CAD build for the part. Positions are in the model's coordinates, mm. Coordinates: 2 decimals unless noted, no trailing zeros. Loops run counter-clockwise (first coordinate to the right, second up) from the corner with the lowest first, then second, coordinate; pieces in that order, holes last. Notation, with made-up numbers: (-15.75, 58.5) -> (3.25, 58.5) arc R21 cw to (3.25, 75.5) -> close; hole circle Ø7 at (32, -40). An arc over 180 degrees is marked (long way). Write each question's results on one line, items separated by ' | '.
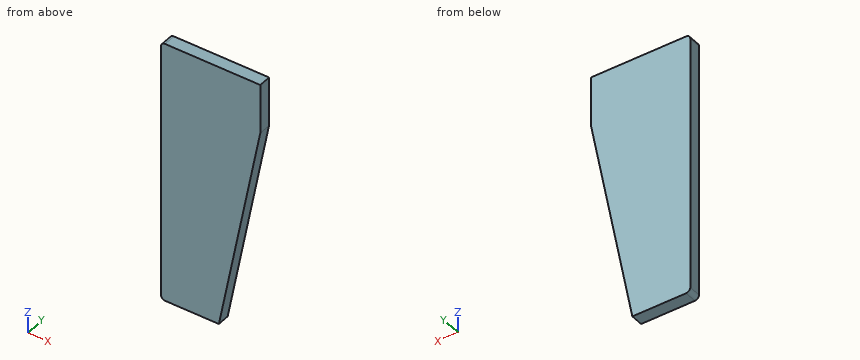
from build123d import *

# Parameters (mm, degrees)
F1_DEPTH = 19.05


with BuildPart() as f1:
    # F0 (on Front) → F1 (new body)
    with BuildSketch(Plane.XZ):
        with BuildLine():
            Line((-233.45189, 237.994913), (-379.50189, 237.994913))
            ThreePointArc((-379.50189, 237.994913), (-383.992018, 236.135041), (-385.85189, 231.644913))
            Line((-385.85189, 231.644913), (-385.85189, -162.055087))
            ThreePointArc((-385.85189, -162.055087), (-383.992018, -166.545215), (-379.50189, -168.405087))
            Line((-379.50189, -168.405087), (-296.95189, -168.405087))
            Line((-296.95189, -168.405087), (-233.45189, 161.794913))
            Line((-233.45189, 161.794913), (-233.45189, 237.994913))
        make_face()
    extrude(amount=F1_DEPTH)


solid = f1.part
1) Slice it at B-B (x = -262). Write the cut outline in (y, z), then the cut area to 3 significant figures.
Outcome:
outline: (-19.05, 13.34) -> (0, 13.34) -> (0, 237.99) -> (-19.05, 237.99) -> close | area: 4,280 mm^2
2) Slice it at C-C (z = 39). Write the cut outline in (x, y).
Outcome:
outline: (-385.85, -19.05) -> (-257.07, -19.05) -> (-257.07, 0) -> (-385.85, 0) -> close
3) Slice it at A-A (y = -12.5). Write the cut outline in (x, z), then the cut area to 3 significant figures.
Outcome:
outline: (-385.85, -162.06) arc R6.35 ccw to (-379.5, -168.41) -> (-296.95, -168.41) -> (-233.45, 161.79) -> (-233.45, 237.99) -> (-379.5, 237.99) arc R6.35 ccw to (-385.85, 231.64) -> close | area: 51,400 mm^2
4) Drill centre lines: L1, parallel to X at y = -7.75, z = 161.5; L2, parallel to X at y = -4.5, z = 139. Where is each one in solid material? Low to high. Write a range as from..to.
Outcome:
L1: x = -385.85..-233.51 | L2: x = -385.85..-237.84
